Could you check a few things on this model? Use its own coordinates, in mm. Face numbers are marked on the shaded views. A direction names the side the tool comes from. Give positions to 0.01 mm unless a question says otherwise; leave off trailing zeros. Order: outer loops, then holes, each group sorted by start corner. A loop starts at its lowest first (then second) coordinate and runs counter-clockwise, first axis right, second up. Notation, with made-up numbers: M 49,28 L 65,28 A10 ccw 65,32 Z; hole C -38,-2 d8. An arc over 180 degrees is marked long. Use a Markdown table: item, result. Add a question column.
```python
from build123d import *

# Parameters (mm, degrees)
SKETCH1_R                = 2.5
BOSS_EXTRUDE1_DEPTH      = 35
BOSS_EXTRUDE1_DEPTH_BACK = 5
SKETCH2_R                = 3.5
BOSS_EXTRUDE2_DEPTH      = 1.5
BOSS_EXTRUDE2_DEPTH_BACK = 1.5
SKETCH3_R                = 1.5
CUT_EXTRUDE1_DEPTH       = 4.5
CUT_EXTRUDE1_DEPTH_BACK  = 4.5
CUT_EXTRUDE2_DEPTH       = 4.5
CUT_EXTRUDE2_DEPTH_BACK  = 4.5


with BuildPart() as part:
    # Sketch1 → Boss-Extrude1 (new body, two sides)
    with BuildSketch(Plane.XY) as boss_extrude1_sk:
        Circle(SKETCH1_R)
    extrude(amount=BOSS_EXTRUDE1_DEPTH)
    extrude(boss_extrude1_sk.sketch, amount=-BOSS_EXTRUDE1_DEPTH_BACK)

    # Sketch2 → Boss-Extrude2 (add, two sides)
    with BuildSketch(Plane.XY) as boss_extrude2_sk:
        Circle(SKETCH2_R)
    extrude(amount=BOSS_EXTRUDE2_DEPTH)
    extrude(boss_extrude2_sk.sketch, amount=-BOSS_EXTRUDE2_DEPTH_BACK)

    # Sketch3 → Cut-Extrude1 (cut, two sides)
    with BuildSketch(Plane(origin=(0, 0, 0), x_dir=(0, 0, -1), z_dir=(1, 0, 0))) as cut_extrude1_sk:
        with Locations((-27.5, 0)):
            Circle(SKETCH3_R)
    extrude(amount=CUT_EXTRUDE1_DEPTH, mode=Mode.SUBTRACT)
    extrude(cut_extrude1_sk.sketch, amount=-CUT_EXTRUDE1_DEPTH_BACK, mode=Mode.SUBTRACT)

    # Sketch4 → Cut-Extrude2 (cut, two sides)
    with BuildSketch(Plane(origin=(0, 0, 0), x_dir=(0, 0, -1), z_dir=(1, 0, 0))) as cut_extrude2_sk:
        Polygon((5, 0), (2, 2.5), (5, 2.5), align=None)
    extrude(amount=CUT_EXTRUDE2_DEPTH, mode=Mode.SUBTRACT)
    extrude(cut_extrude2_sk.sketch, amount=-CUT_EXTRUDE2_DEPTH_BACK, mode=Mode.SUBTRACT)


solid = part.part
```
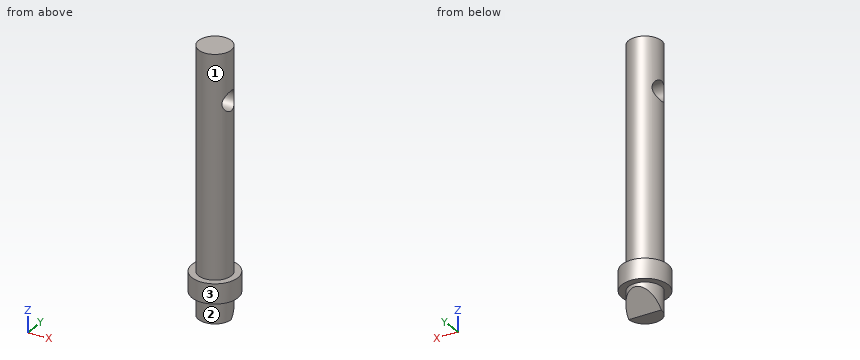
1) Suppose I cut it at D-D on z = 6. Please give me the cut outline in (x, y).
2) Suppose I cut it at A-A on x = 0. Please give me the cut outline in (y, z).
3) For pin 1 (4 mm diameter, centred on y = 0, z = 27.5, fed in from -X); pin 2 (1 mm diameter, centred on y = 0, z = 18, fed in from +X); pin 3 (3 mm diameter, centred on x = -1, z = 19.5, fed in from -Y), each with a flat end and sliding along its axis, tell me the tip position at first contact or that it passes through.
4) Please list where these lines run through material, in increasing order: line 1 (Z direction, x = -3, y = 1.5); line 2 (Y direction, x = 0.5, z = 27.5). Write a range as from..to.
5) Suppose I cut it at C-C on z = 27.5. Please give me the cut outline in (x, y).
6) Suppose I cut it at B-B on y = 1. Please give me the cut outline in (x, z).
7) For the marked faces 1, 2 and 3, which set-ups out of +Z, -Z, +X, -X, +Y, -Y let a thin tool reach every point of the face, with its end or its side?
Values found:
| question | item | result |
|---|---|---|
| 1 | outline | C 0,0 d5 |
| 2 | outline | M -3.5,-1.5 L -2.5,-1.5 L -2.5,-5 L 0,-5 L 2.5,-2 L 2.5,-1.5 L 3.5,-1.5 L 3.5,1.5 L 2.5,1.5 L 2.5,35 L -2.5,35 L -2.5,1.5 L -3.5,1.5 Z; hole C 0,27.5 d3 |
| 3 | pin 1 | stops at x = -2.5 |
| 3 | pin 2 | stops at x = 2.5 |
| 3 | pin 3 | stops at y = -2.5 |
| 4 | line 1 | z = -1.5..1.5 |
| 4 | line 2 | y = -2.45..-1.5, 1.5..2.45 |
| 5 | outline | M -2,-1.5 A2.5 ccw 2,-1.5 Z; M -2,1.5 L 2,1.5 A2.5 ccw Z |
| 6 | outline | M -3.35,-1.5 L -2.29,-1.5 L -2.29,-3.8 L 2.29,-3.8 L 2.29,-1.5 L 3.35,-1.5 L 3.35,1.5 L 2.29,1.5 L 2.29,26.38 L -2.29,26.38 L -2.29,1.5 L -3.35,1.5 Z; M -2.29,28.62 L 2.29,28.62 L 2.29,35 L -2.29,35 Z |
| 7 | face 1 | +Z |
| 7 | face 2 | -Z |
| 7 | face 3 | +Z, -Z |
